Autodesk Inventor part; units mm, degrees
ref_plane "YZ Plane" through (0, 0, 0) normal (1, 0, 0) x (0, 1, 0)
ref_plane "XZ Plane" through (0, 0, 0) normal (0, 1, 0) x (-1, 0, 0)
ref_plane "XY Plane" through (0, 0, 0) normal (0, 0, 1) x (1, 0, 0)
sketch "Sketch1" plane through (0, 0, 0) normal (0, 0, 1) x (1, 0, 0)
  line L0 (0, 100) -> (0, 50) construction
  line L1 (0, 47) -> (0, 0) construction
  line L2 (0, 50) -> (0, 47) construction
  arc A0 (42, -1970) -> (25, 0) centre (-10972.0978, -1079.9722) ccw
  line L3 (42, -1970) -> (0, -1970)
  line L4 (0, -1970) -> (0, 0)
  line L5 (0, 0) -> (25, 0)
  line L6 (21, 0) -> (41.9305, -240)
  line L7 (41.9305, -240) -> (45.9305, -240)
  dimension "d115" = 3
  dimension "d131" = 11050
  dimension "d132" = 25
  dimension "d133" = 42
  dimension "d134" = 1970
  dimension "d145" = 4
  dimension "d146" = 240
  dimension "d147" = 4
extrude "Plate3" add sketch "Sketch1" along normal blind 3 contours L3 L4 L5 L6 L7 A0
sketch "Sketch3" plane through (0, 0, 0) normal (0, 0, -1) x (-1, 0, 0)
  line L0 (0, 0) -> (0, -1970) construction
  line L1 (-21, 0) -> (0, 0) construction
  arc A0 (-45.9305, -240) -> (-42, -1970) centre (10972.0978, -1079.9722) ccw construction
  line L2 (0, -1970) -> (-42, -1970)
  circle A1 centre (-15, -600) radius 5.5
  line L3 (-41.9305, -240) -> (-21, 0)
  line L4 (-45.9305, -240) -> (-41.9305, -240)
  circle A2 centre (-15, -680) radius 5.5
  circle A3 centre (-37.5699, -190) radius 15
  circle A4 centre (-15, -1800) radius 5.5
  circle A5 centre (-15, -1880) radius 5.5
  circle A6 centre (-15, -1200) radius 5.5
  circle A7 centre (-15, -1280) radius 5.5
  dimension "d135" = 11
  dimension "d136" = 15
  dimension "d148" = 600
  dimension "d149" = 80
  dimension "d150" = 30
  dimension "d151" = 190
  dimension "d153" = 80
  dimension "d154" = 1200
  dimension "d157" = 80
  dimension "d159" = 1200
extrude "Cut1" cut sketch "Sketch3" against normal blind 3
equation "\"BendReliefWidth\" = Thickness"
equation "\"BendReliefDepth\" = 0.5 * Thickness"
equation "\"CornerReliefSize\" = 4 * Thickness"
equation "\"MinimumRemnant\" = 2 * Thickness"
equation "\"GapSize\" = Thickness"
properties part number "MSC 814 wall inner rib" material "AISI304"
Could you check a few things on this model? Use its own coordinates, in mm. Coordinates: 2 decimals unless noted, no trailing zeros. Write each loop counter-clockwise with the first axis right and the second up, starting at its lowest first coordinate (ties: lowest second). Pieces come first, ordered by that corner, then holes. Notation, with made-up numbers: M 5.5,29 L 35.5,29 A14 ccw 35.5,38 Z; hole C 35.25,-1 d5. An arc over 180 degrees is marked long. One line per question, with ' | ' between items.
1) If we mould it in two halves opening along Y, with no side actions, what happens to faces 1 (the face through (30, -971, 3)), 2 (the face through (77.895, -1092.955, 1.479))? For each: released by +Y, released by -Y, zero draft, split by the parting line, or undercut.
Checks:
face 1: zero draft | face 2: split by the parting line
2) I need wall thicknesses on probe 1 along Y at (x, z) = (37, 2.6); probe 2 along X at (y, z) = (-600, 1.1); probe 3 along X at (y, z) = (-675, 0.6). Which ranges of each line are inside material? Lowest first, please. Write a range as [from, to].
Checks:
probe 1: [-1970, -204.99] | probe 2: [0, 9.5], [20.5, 67.47] | probe 3: [0, 12.71], [17.29, 70.48]
3) For pin 1 Ø14.5 at (x, y) = (15, -1200) entering from -Z; pin 2 Ø1.5 at (x, z) = (37.5, 2) entering from +Y; pin 3 Ø9 at (x, y) = (15, -1880) entering from -Z, each with a flat end and sliding along its axis, tell me the tip position at first contact or that it passes through.
Checks:
pin 1: z = 0 | pin 2: y = -204.98 | pin 3: through
4) Imagine slicing it at C-C, the plane y = -542.5. Write out the boundary of the cut face in (x, z), and give its area (3 significant figures).
Checks:
outline: M 0,0 L 64.82,0 L 64.82,3 L 0,3 Z | area: 194 mm²
5) Imagine slicing it at A-A, the plane z = 1.9. Write out the boundary of the cut face in (x, y).
Checks:
outline: M 0,-1970 L 42,-1970 A11050 ccw 45.93,-240 L 41.93,-240 L 38.87,-204.94 A15 cw 36.27,-175.06 L 21,0 L 0,0 Z; hole C 15,-1880 d11; hole C 15,-1800 d11; hole C 15,-1280 d11; hole C 15,-1200 d11; hole C 15,-680 d11; hole C 15,-600 d11
6) Imagine slicing it at B-B, the plane y = -795. Write out the boundary of the cut face in (x, z).
Checks:
outline: M 0,0 L 74.23,0 L 74.23,3 L 0,3 Z
